Read the model definition and answer for the solid it produces. Units are mm, in the model's axes. Coordinates: 2 decimals unless noted, no trailing zeros. Write each loop counter-clockwise with the first axis right and the second up, starting at its lowest first coordinate (ties: lowest second). Pieces come first, ordered by that corner, then holes. Notation, with made-up numbers: M 4,81.25 L 55,81.25 A18 ccw 55,102.25 Z; hole C -25.75,26.5 d1. An arc over 180 degrees is marked long. Write item = value, one per line.
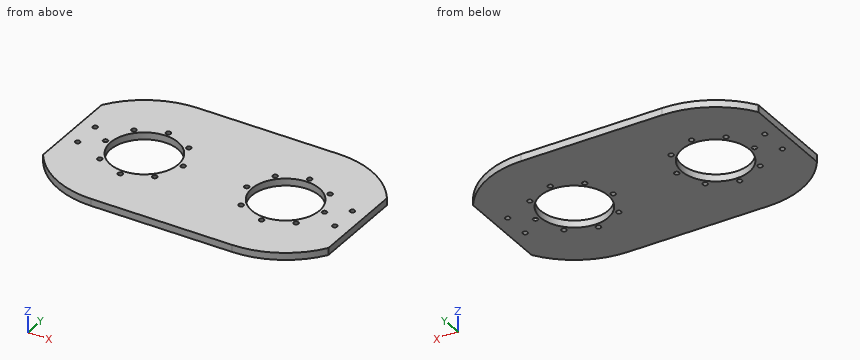
from build123d import *

# Parameters (mm, degrees)
EXTRUDE_1_DEPTH          = 5
SKETCH_2_R               = 24
CUT_EXTRUDE_1_DEPTH      = 6
HOLE_WIZARD_M3_1_D       = 3.4
PATTERN_CIRCULAR_1_COUNT = 8
MIRROR_1_COPY_1_D        = 3.4
MIRROR_1_COPY_2_D        = 3.4
MIRROR_1_COPY_3_D        = 3.4
MIRROR_1_COPY_4_D        = 3.4
MIRROR_1_COPY_5_D        = 3.4
MIRROR_1_COPY_6_D        = 3.4
MIRROR_1_COPY_7_D        = 3.4
CUT_EXTRUDE_2_DEPTH      = 6
HOLE_WIZARD_M3_2_D       = 3.4


with BuildPart() as part:
    # ｽｹｯﾁ1 → ﾎﾞｽ - 押し出し1 (new body)
    with BuildSketch(Plane.XY):
        with BuildLine():
            Line((-50, 61), (50, 61))
            ThreePointArc((50, 61), (111, 0), (50, -61))
            Line((50, -61), (-50, -61))
            ThreePointArc((-50, -61), (-111, 0), (-50, 61))
        make_face()
    extrude(amount=EXTRUDE_1_DEPTH)

    # ｽｹｯﾁ2 → ｶｯﾄ - 押し出し1 (cut, through all)
    with BuildSketch(Plane.XY.offset(5)):
        with Locations((-50, 0)):
            Circle(SKETCH_2_R)
    cut_extrude_1 = extrude(amount=-CUT_EXTRUDE_1_DEPTH, mode=Mode.SUBTRACT)

    # M3 すきま穴1 (through all)
    with Locations(Plane.XY.offset(5)):
        with Locations((-50, 27.5)):
            hole_wizard_m3_1 = Hole(HOLE_WIZARD_M3_1_D / 2)

    # 円形ﾊﾟﾀｰﾝ1: M3 すきま穴1 ×8 about axis
    pattern_circular_1_axis = Axis((-50, 0, 0), (0, 0, 1))
    for i in range(1, PATTERN_CIRCULAR_1_COUNT):
        add(hole_wizard_m3_1.rotate(pattern_circular_1_axis, i * 360 / PATTERN_CIRCULAR_1_COUNT), mode=Mode.SUBTRACT)

    # ﾐﾗｰ1: ｶｯﾄ - 押し出し1, M3 すきま穴1 across plane
    add(cut_extrude_1.mirror(Plane(origin=(0, 0, 0), x_dir=(0, 0, 1), z_dir=(1, 0, 0))), mode=Mode.SUBTRACT)
    add(hole_wizard_m3_1.mirror(Plane(origin=(0, 0, 0), x_dir=(0, 0, 1), z_dir=(1, 0, 0))), mode=Mode.SUBTRACT)

    # ﾐﾗｰ1 copy 1 (through all)
    with Locations(Plane(origin=(14.644660941, 35.355339059, 5), x_dir=(-0.707106781, 0.707106781, 0), z_dir=(0, 0, 1))):
        with Locations((-50, -27.5)):
            Hole(MIRROR_1_COPY_1_D / 2)

    # ﾐﾗｰ1 copy 2 (through all)
    with Locations(Plane(origin=(50, 50, 5), x_dir=(0, 1, 0), z_dir=(0, 0, 1))):
        with Locations((-50, -27.5)):
            Hole(MIRROR_1_COPY_2_D / 2)

    # ﾐﾗｰ1 copy 3 (through all)
    with Locations(Plane(origin=(85.355339059, 35.355339059, 5), x_dir=(0.707106781, 0.707106781, 0), z_dir=(0, 0, 1))):
        with Locations((-50, -27.5)):
            Hole(MIRROR_1_COPY_3_D / 2)

    # ﾐﾗｰ1 copy 4 (through all)
    with Locations(Plane(origin=(100, 0, 5), x_dir=(1, 0, 0), z_dir=(0, 0, 1))):
        with Locations((-50, -27.5)):
            Hole(MIRROR_1_COPY_4_D / 2)

    # ﾐﾗｰ1 copy 5 (through all)
    with Locations(Plane(origin=(85.355339059, -35.355339059, 5), x_dir=(0.707106781, -0.707106781, 0), z_dir=(0, 0, 1))):
        with Locations((-50, -27.5)):
            Hole(MIRROR_1_COPY_5_D / 2)

    # ﾐﾗｰ1 copy 6 (through all)
    with Locations(Plane(origin=(50, -50, 5), x_dir=(0, -1, 0), z_dir=(0, 0, 1))):
        with Locations((-50, -27.5)):
            Hole(MIRROR_1_COPY_6_D / 2)

    # ﾐﾗｰ1 copy 7 (through all)
    with Locations(Plane(origin=(14.644660941, -35.355339059, 5), x_dir=(-0.707106781, -0.707106781, 0), z_dir=(0, 0, 1))):
        with Locations((-50, -27.5)):
            Hole(MIRROR_1_COPY_7_D / 2)

    # ｽｹｯﾁ5 → ｶｯﾄ - 押し出し2 (cut, through all)
    with BuildSketch(Plane.XY.offset(5)):
        with BuildLine():
            Line((-101, 33.466401061), (-101, -33.466401061))
            ThreePointArc((-101, -33.466401061), (-111, 0), (-101, 33.466401061))
        make_face()
    cut_extrude_2 = extrude(amount=-CUT_EXTRUDE_2_DEPTH, mode=Mode.SUBTRACT)

    # M3 すきま穴2 (through all)
    with Locations(Plane.XY.offset(5)):
        with Locations((-91, 10), (-91, -10)):
            hole_wizard_m3_2 = Hole(HOLE_WIZARD_M3_2_D / 2)

    # ﾐﾗｰ2: ｶｯﾄ - 押し出し2, M3 すきま穴2 across plane
    add(cut_extrude_2.mirror(Plane(origin=(0, 0, 0), x_dir=(0, 0, 1), z_dir=(1, 0, 0))), mode=Mode.SUBTRACT)
    add(hole_wizard_m3_2.mirror(Plane(origin=(0, 0, 0), x_dir=(0, 0, 1), z_dir=(1, 0, 0))), mode=Mode.SUBTRACT)


solid = part.part
Item 1: Find section A-A (x = -34.5). Determine the outline of the cut face in (y, z), and give its area (3 significant figures).
Worked answers:
outline = M -61,0 L -18.32,0 L -18.32,5 L -61,5 Z; M 18.32,0 L 61,0 L 61,5 L 18.32,5 Z
area = 427 mm²
Item 2: Find section C-C (y = 38.5). Determine the outline of the cut face in (x, z), and give its area (3 significant figures).
Worked answers:
outline = M -97.32,0 L 97.32,0 L 97.32,5 L -97.32,5 Z
area = 973 mm²
Item 3: Find section B-B (z = 3.2). State how many separate pieces and enclosed holes the cut face has, and give its area (3 significant figures).
Worked answers:
separate_pieces = 1
enclosed_holes = 22
area = 19,200 mm²
Item 4: Consider line 1 along Y through (x, z) = (50, 1.45); line 2 along Y through (x, z) = (-91, 1.25); line 3 along X through (y, z) = (-7, 2.1). Determine where each line is inside the solid, lowest interval first. Write a range as from..to.
Worked answers:
line_1 = -61..-29.2, -25.8..-24, 24..25.8, 29.2..61
line_2 = -45.17..-11.7, -8.3..8.3, 11.7..45.17
line_3 = -101..-72.96, -27.04..27.04, 72.96..101
